CAD build for the part. Positions are in the model's coordinates, mm. Face numbers are marked on the shaded views. A direction names the side the tool comes from. Coordinates: 2 decimals unless noted, no trailing zeros. Loops run counter-clockwise (first coordinate to the right, second up) from the corner with the lowest first, then second, coordinate; pieces in that order, holes last.
1) Saw through at B-B, the plane x = -104.5. Write the cut outline in (y, z).
2) Wall check: line 1 along X through (y, z) = (76, 122); line 2 along X through (y, z) = (38, -70.5); line 3 along Y through (x, z) = (111.7, 125). Give the ranges that are in metal, low to high.
3) Saw through at A-A, the plane z = 0. Write the cut outline in (x, y).
4) Pin check, flat tips, straight feed: pin 1 Ø5.5 at (y, z) = (15, -125) entering from -X (1 decimal); pin 2 Ø10 at (x, z) = (-58.5, -43.5) entering from +Y; pin 3 Ø2 at (x, y) = (45.5, 2) entering from +Z; pin 4 Ø4.5 at (x, z) = (109, 58.5) entering from +Y. Stop position of each tip, or through.
5) Saw through at C-C, the plane y = 44.5. Give the number of separate pieces and of enclosed holes in the cut face, and give its area (3 significant figures).
6) Which spindle directions (+Z, -Z, +X, -X, +Y, -Y) get a long thin tool onto all of the face, cutting with end or side? Do the marked faces 5, 6, 7, 8 and 9. Say none if no direction does.
7) Two-plate mould, pull along Z, no slides. Class the marked faces 1, 2, 3 and 4: +Z half, -Z half, draft (parallel to the pull), parting line (faces both ways), or undercut.
```python
from build123d import *

# Parameters (mm, degrees)
SKETCH_1_W                = 290
SKETCH_1_H                = 290
EXTRUDE_1_DEPTH           = 4
EXTRUDE_2_DEPTH           = 76
SKETCH_16_W               = 130
SKETCH_16_H               = 50
CUT_EXTRUDE_11_DEPTH      = 10
SKETCH_4_W                = 6
SKETCH_4_H                = 290
EXTRUDE_3_DEPTH           = 76
SKETCH_7_R                = 2
CUT_EXTRUDE_3_DEPTH       = 10
SKETCH_14_W               = 80
SKETCH_14_H               = 30
CUT_EXTRUDE_9_DEPTH       = 20
CUT_EXTRUDE_10_DEPTH      = 334.95358959
CUT_EXTRUDE_10_DEPTH_BACK = 334.95358959
SKETCH_15_R               = 3.5
FILLET_1_R                = 5
CUT_EXTRUDE_12_DEPTH      = 292.590466236
CUT_EXTRUDE_12_DEPTH_BACK = 292.590466236
SKETCH_17_R               = 19.5
SKETCH_17_R_2             = 3
SKETCH_18_W               = 4
SKETCH_18_H               = 190
EXTRUDE_4_DEPTH           = 20
CHAMFER_1_SIZE            = 40
CUT_EXTRUDE_13_DEPTH      = 334.95358959
CUT_EXTRUDE_13_DEPTH_BACK = 334.95358959
FILLET_2_R                = 5


with BuildPart() as part:
    # Эскиз1 → Бобышка-Вытянуть1 (new body)
    with BuildSketch(Plane(origin=(0, 0, 0), x_dir=(1, 0, 0), z_dir=(0, 1, 0))):
        Rectangle(SKETCH_1_W, SKETCH_1_H)
    extrude(amount=EXTRUDE_1_DEPTH)

    # Эскиз2 → Бобышка-Вытянуть2 (add)
    with BuildSketch(Plane(origin=(0, 4, 0), x_dir=(1, 0, 0), z_dir=(0, 1, 0))):
        Polygon((145, 145), (109, 145), (109, 95), (-21, 95), (-21, 145), (-139, 145), (-139, 139), (-27, 139), (-27, 89), (115, 89), (115, 139), (139, 139), (139, -139), (115, -139), (115, -89), (-27, -89), (-27, -139), (-139, -139), (-139, -145), (-21, -145), (-21, -95), (109, -95), (109, -145), (145, -145), (145, 0.239524614), align=None)
    extrude(amount=EXTRUDE_2_DEPTH)

    # Эскиз16 → Вырез-Вытянуть11 (cut)
    with BuildSketch(Plane(origin=(0, 4, 0), x_dir=(1, 0, 0), z_dir=(0, 1, 0))):
        with Locations((44, 120)):
            Rectangle(SKETCH_16_W, SKETCH_16_H)
        with Locations((44, -120)):
            Rectangle(SKETCH_16_W, SKETCH_16_H)
    extrude(amount=-CUT_EXTRUDE_11_DEPTH, mode=Mode.SUBTRACT)

    # Эскиз4 → Бобышка-Вытянуть3 (add)
    with BuildSketch(Plane(origin=(0, 4, 0), x_dir=(1, 0, 0), z_dir=(0, 1, 0))):
        with Locations((-142, 0)):
            Rectangle(SKETCH_4_W, SKETCH_4_H)
    extrude(amount=EXTRUDE_3_DEPTH)

    # Эскиз7 → Вырез-Вытянуть3 (cut)
    with BuildSketch(Plane(origin=(0, 4, 0), x_dir=(1, 0, 0), z_dir=(0, 1, 0))):
        with Locations(Location((119, 82, 0), (0, 0, 270))):
            Circle(SKETCH_7_R)
        with Locations(Location((126, 75, 0), (0, 0, 270))):
            Circle(SKETCH_7_R)
        with Locations(Location((-31, 82, 0), (0, 0, 270))):
            Circle(SKETCH_7_R)
        with Locations(Location((-38, 75, 0), (0, 0, 270))):
            Circle(SKETCH_7_R)
        with Locations(Location((119, -82, 0), (0, 0, 270))):
            Circle(SKETCH_7_R)
        with Locations(Location((126, -75, 0), (0, 0, 270))):
            Circle(SKETCH_7_R)
        with Locations(Location((-38, -75, 0), (0, 0, 270))):
            Circle(SKETCH_7_R)
        with Locations(Location((-31, -82, 0), (0, 0, 270))):
            Circle(SKETCH_7_R)
    extrude(amount=-CUT_EXTRUDE_3_DEPTH, mode=Mode.SUBTRACT)

    # Эскиз14 → Вырез-Вытянуть9 (cut)
    with BuildSketch(Plane(origin=(0, 4, 0), x_dir=(1, 0, 0), z_dir=(0, 1, 0))):
        with Locations((44, 70)):
            Rectangle(SKETCH_14_W, SKETCH_14_H)
        with Locations((44, -70)):
            Rectangle(SKETCH_14_W, SKETCH_14_H)
    extrude(amount=-CUT_EXTRUDE_9_DEPTH, mode=Mode.SUBTRACT)

    # Эскиз15 → Вырез-Вытянуть10 (cut, two sides: drawn at the far end of the back side and taken through both)
    with BuildSketch(Plane.ZY.offset(145).offset(-CUT_EXTRUDE_10_DEPTH_BACK)):
        with Locations((0, 65)):
            Circle(SKETCH_15_R)
        with Locations((125, 65)):
            Circle(SKETCH_15_R)
        with Locations((-125, 65)):
            Circle(SKETCH_15_R)
        with Locations((-125, 15)):
            Circle(SKETCH_15_R)
        with Locations((125, 15)):
            Circle(SKETCH_15_R)
        with Locations((0, 15)):
            Circle(SKETCH_15_R)
    extrude(amount=CUT_EXTRUDE_10_DEPTH + CUT_EXTRUDE_10_DEPTH_BACK, mode=Mode.SUBTRACT)

    # Скругление1
    fillet_1_edges = [part.edges().sort_by_distance(p)[0] for p in [
        (109, 40, -145),
        (109, 40, -95),
        (-21, 40, -95),
        (-21, 40, -145),
        (-139, 42, -139),
        (-27, 42, -139),
        (-27, 42, -89),
        (115, 42, -89),
        (115, 42, -139),
        (139, 42, -139),
        (139, 42, 139),
        (115, 42, 139),
        (115, 42, 89),
        (-27, 42, 89),
        (-27, 42, 139),
        (-139, 42, 139),
        (-21, 40, 145),
        (-21, 40, 95),
        (109, 40, 95),
        (109, 40, 145),
    ]]
    fillet(fillet_1_edges, radius=FILLET_1_R)

    # Эскиз17 → Вырез-Вытянуть12 (cut, two sides: drawn at the far end of the back side and taken through both)
    with BuildSketch(Plane.XY.offset(95).offset(-CUT_EXTRUDE_12_DEPTH_BACK)):
        with Locations((44, 33)):
            Circle(SKETCH_17_R)
        with Locations((20.45, 56.55)):
            Circle(SKETCH_17_R_2)
        with Locations((67.55, 56.55)):
            Circle(SKETCH_17_R_2)
        with Locations((67.55, 9.45)):
            Circle(SKETCH_17_R_2)
        with Locations((20.45, 9.45)):
            Circle(SKETCH_17_R_2)
    extrude(amount=CUT_EXTRUDE_12_DEPTH + CUT_EXTRUDE_12_DEPTH_BACK, mode=Mode.SUBTRACT)

    # Эскиз18 → Бобышка-Вытянуть4 (add)
    with BuildSketch(Plane(origin=(0, 4, 0), x_dir=(1, 0, 0), z_dir=(0, 1, 0))):
        with Locations((-21, 0)):
            Rectangle(SKETCH_18_W, SKETCH_18_H)
        with Locations((109, 0)):
            Rectangle(SKETCH_18_W, SKETCH_18_H)
    extrude(amount=EXTRUDE_4_DEPTH)

    # Фаска1
    chamfer_1_edges = [part.edges().sort_by_distance(p)[0] for p in [
        (-22.50254481, 24, -89.025319235),
        (-20.5, 24, 89),
        (-20.5, 24, -89),
        (-22.50254481, 24, 89.025319235),
        (110.50254481, 24, -89.025319235),
        (110.50254481, 24, 89.025319235),
        (108.5, 24, 89),
        (108.5, 24, -89),
    ]]
    chamfer(chamfer_1_edges, length=CHAMFER_1_SIZE)

    # Эскиз19 → Вырез-Вытянуть13 (cut, two sides: drawn at the far end of the back side and taken through both)
    with BuildSketch(Plane(origin=(145, 0, 0), x_dir=(0, 0, -1), z_dir=(1, 0, 0)).offset(-CUT_EXTRUDE_13_DEPTH_BACK)):
        Polygon((-65, 30), (65, 30), (89, 80), (-89, 80), align=None)
    extrude(amount=CUT_EXTRUDE_13_DEPTH + CUT_EXTRUDE_13_DEPTH_BACK, mode=Mode.SUBTRACT)

    # Скругление2
    fillet_2_edges = [part.edges().sort_by_distance(p)[0] for p in [
        (84, 2, -85),
        (84, 2, -55),
        (4, 2, -55),
        (4, 2, -85),
        (4, 2, 85),
        (4, 2, 55),
        (84, 2, 55),
        (84, 2, 85),
        (-19, 34, 89),
        (-19, 34, -89),
        (107, 34, 89),
        (107, 34, -89),
    ]]
    fillet(fillet_2_edges, radius=FILLET_2_R)


solid = part.part
```
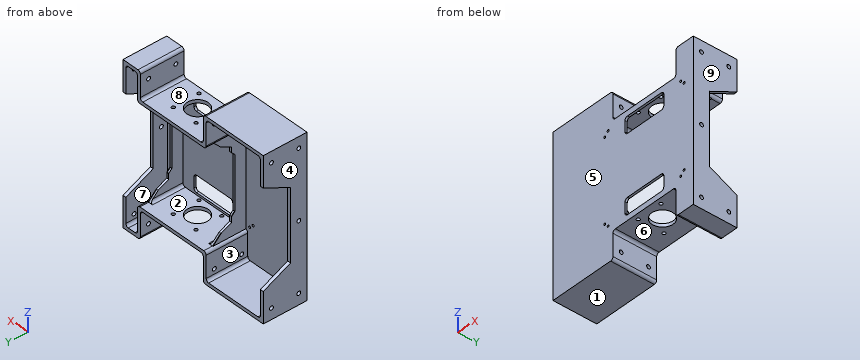
Data:
1. outline: (0, -145) - (80, -145) - (80, -139) - (4, -139) - (4, 139) - (80, 139) - (80, 145) - (0, 145) - close
2. line 1: x = -145 to -139, -27 to -21, 109 to 115, 139 to 145
2. line 2: x = -145 to -139, -23 to -19, 107 to 111, 139 to 145
2. line 3: y = 0 to 11.5, 18.5 to 61.5, 68.5 to 80
3. outline: (-145, 0) - (145, 0) - (145, 11.5) - (139, 11.5) - (139, 4) - (111, 4) - (111, 24) - (107, 24) - (107, 4) - (-19, 4) - (-19, 24) - (-23, 24) - (-23, 4) - (-139, 4) - (-139, 11.5) - (-145, 11.5) - close; (-145, 18.5) - (-139, 18.5) - (-139, 30) - (-145, 30) - close; (139, 18.5) - (145, 18.5) - (145, 30) - (139, 30) - close
4. pin 1: passes through
4. pin 2: stops at y = 4
4. pin 3: stops at z = 95
4. pin 4: stops at y = 30
5. separate pieces: 4
5. enclosed holes: 0
5. area: 6,230 mm2
6. face 5: +Z, -Z, +X, -X, -Y
6. face 6: -Z, +Y, -Y
6. face 7: +Y
6. face 8: +Z, +Y, -Y
6. face 9: +Z, -Z, +X, +Y, -Y
7. face 1: -Z half
7. face 2: undercut
7. face 3: undercut
7. face 4: draft
